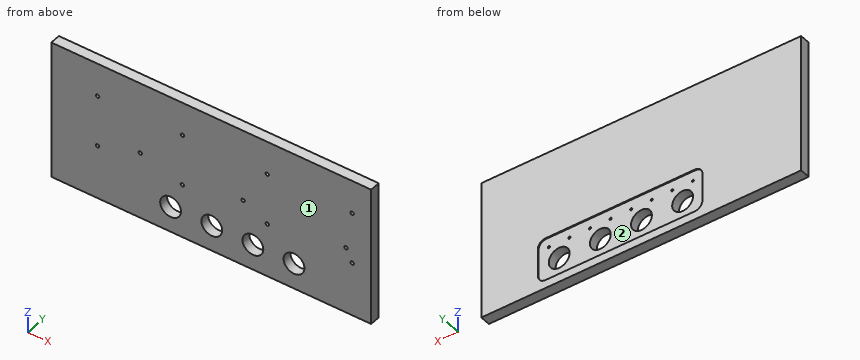
```python
from build123d import *

# Parameters (mm, degrees)
SKETCH_1_W          = 622
SKETCH_1_H          = 270
EXTRUDE_1_DEPTH     = 20
SKETCH_2_W          = 320
SKETCH_2_H          = 84
CUT_EXTRUDE_1_DEPTH = 2
CUT_EXTRUDE_2_REACH = 341.514
SKETCH_3_R          = 20.25
SKETCH_4_R          = 2.1
SKETCH_4_R_2        = 20.25
CUT_EXTRUDE_3_DEPTH = 10
FILLET_1_R          = 15
SKETCH_5_R          = 3.35
CUT_EXTRUDE_4_DEPTH = 12


with BuildPart() as part:
    # 草图1 → 凸台-拉伸1 (new body)
    with BuildSketch(Plane(origin=(0, 0, 0), x_dir=(1, 0, 0), z_dir=(0, 1, 0))):
        Rectangle(SKETCH_1_W, SKETCH_1_H)
    extrude(amount=EXTRUDE_1_DEPTH)

    # 草图2 → 切除-拉伸1 (cut)
    with BuildSketch(Plane(origin=(0, 20, 0), x_dir=(1, 0, 0), z_dir=(0, 1, 0))):
        with Locations((41, 77)):
            Rectangle(SKETCH_2_W, SKETCH_2_H)
    extrude(amount=-CUT_EXTRUDE_1_DEPTH, mode=Mode.SUBTRACT)

    # 草图3 → 切除-拉伸2 (cut, up to next)
    with BuildSketch(Plane(origin=(0, 18, 0), x_dir=(1, 0, 0), z_dir=(0, 1, 0)), mode=Mode.PRIVATE) as cut_extrude_2_sk1:
        with Locations(Location((-79, 85, 0), (0, 0, 270))):
            Circle(SKETCH_3_R)
    cut_extrude_2_tool1 = extrude(cut_extrude_2_sk1.sketch, amount=-CUT_EXTRUDE_2_REACH, mode=Mode.PRIVATE) & part.part
    # 草图3 → 切除-拉伸2 (cut, up to next)
    with BuildSketch(Plane(origin=(0, 18, 0), x_dir=(1, 0, 0), z_dir=(0, 1, 0)), mode=Mode.PRIVATE) as cut_extrude_2_sk2:
        with Locations(Location((1, 85, 0), (0, 0, 270))):
            Circle(SKETCH_3_R)
    cut_extrude_2_tool2 = extrude(cut_extrude_2_sk2.sketch, amount=-CUT_EXTRUDE_2_REACH, mode=Mode.PRIVATE) & part.part
    # 草图3 → 切除-拉伸2 (cut, up to next)
    with BuildSketch(Plane(origin=(0, 18, 0), x_dir=(1, 0, 0), z_dir=(0, 1, 0)), mode=Mode.PRIVATE) as cut_extrude_2_sk3:
        with Locations(Location((81, 85, 0), (0, 0, 270))):
            Circle(SKETCH_3_R)
    cut_extrude_2_tool3 = extrude(cut_extrude_2_sk3.sketch, amount=-CUT_EXTRUDE_2_REACH, mode=Mode.PRIVATE) & part.part
    # 草图3 → 切除-拉伸2 (cut, up to next)
    with BuildSketch(Plane(origin=(0, 18, 0), x_dir=(1, 0, 0), z_dir=(0, 1, 0)), mode=Mode.PRIVATE) as cut_extrude_2_sk4:
        with Locations(Location((161, 85, 0), (0, 0, 270))):
            Circle(SKETCH_3_R)
    cut_extrude_2_tool4 = extrude(cut_extrude_2_sk4.sketch, amount=-CUT_EXTRUDE_2_REACH, mode=Mode.PRIVATE) & part.part
    add(cut_extrude_2_tool1.solids().sort_by_distance((-79, 18, -85))[0], mode=Mode.SUBTRACT)
    add(cut_extrude_2_tool2.solids().sort_by_distance((1, 18, -85))[0], mode=Mode.SUBTRACT)
    add(cut_extrude_2_tool3.solids().sort_by_distance((81, 18, -85))[0], mode=Mode.SUBTRACT)
    add(cut_extrude_2_tool4.solids().sort_by_distance((161, 18, -85))[0], mode=Mode.SUBTRACT)

    # 草图4 → 切除-拉伸3 (cut)
    with BuildSketch(Plane(origin=(0, 18, 0), x_dir=(1, 0, 0), z_dir=(0, 1, 0))):
        with Locations(Location((-99, 54, 0), (0, 0, 270))):
            Circle(SKETCH_4_R)
        with Locations(Location((-79, 85, 0), (0, 0, 270))):
            Circle(SKETCH_4_R_2)
        with Locations(Location((-59, 54, 0), (0, 0, 270))):
            Circle(SKETCH_4_R)
        with Locations(Location((-19, 54, 0), (0, 0, 270))):
            Circle(SKETCH_4_R)
        with Locations(Location((21, 54, 0), (0, 0, 270))):
            Circle(SKETCH_4_R)
        with Locations(Location((61, 54, 0), (0, 0, 270))):
            Circle(SKETCH_4_R)
        with Locations(Location((101, 54, 0), (0, 0, 270))):
            Circle(SKETCH_4_R)
        with Locations(Location((141, 54, 0), (0, 0, 270))):
            Circle(SKETCH_4_R)
        with Locations(Location((181, 54, 0), (0, 0, 270))):
            Circle(SKETCH_4_R)
    extrude(amount=-CUT_EXTRUDE_3_DEPTH, mode=Mode.SUBTRACT)

    # 圆角1
    fillet_1_edges = [part.edges().sort_by_distance(p)[0] for p in [
        (-119, 19, -35),
        (-119, 19, -119),
        (201, 19, -119),
        (201, 19, -35),
    ]]
    fillet(fillet_1_edges, radius=FILLET_1_R)

    # 草图5 → 切除-拉伸4 (cut)
    with BuildSketch(Plane.XZ):
        with Locations(Location((274, -30, 0), (0, 0, 270))):
            Circle(SKETCH_5_R)
        with Locations(Location((262, -5, 0), (0, 0, 270))):
            Circle(SKETCH_5_R)
        with Locations(Location((109, -30, 0), (0, 0, 270))):
            Circle(SKETCH_5_R)
        with Locations(Location((-56, -30, 0), (0, 0, 270))):
            Circle(SKETCH_5_R)
        with Locations(Location((-221, -30, 0), (0, 0, 270))):
            Circle(SKETCH_5_R)
        with Locations(Location((-138, -5, 0), (0, 0, 270))):
            Circle(SKETCH_5_R)
        with Locations(Location((62, -5, 0), (0, 0, 270))):
            Circle(SKETCH_5_R)
        with Locations(Location((274, 70, 0), (0, 0, 270))):
            Circle(SKETCH_5_R)
        with Locations(Location((109, 70, 0), (0, 0, 270))):
            Circle(SKETCH_5_R)
        with Locations(Location((-56, 70, 0), (0, 0, 270))):
            Circle(SKETCH_5_R)
        with Locations(Location((-221, 70, 0), (0, 0, 270))):
            Circle(SKETCH_5_R)
    extrude(amount=-CUT_EXTRUDE_4_DEPTH, mode=Mode.SUBTRACT)


solid = part.part
```
Check sheet for the modelled part. Datum: model origin and axes. Units: mm. Face numbers are marked on the shaded views. Coordinates: 2 decimals unless noted, no trailing zeros. Write each loop counter-clockwise with the first axis right and the second up, starting at its lowest first coordinate (ties: lowest second). Pieces come first, ordered by that corner, then holes. Notation, with made-up numbers: M 38,51.25 L 55,51.25 A17 cw 55,74.25 Z; hole C 51,63.5 d8. An arc over 180 degrees is marked long. Use one line per item in the form item = value.
Item 1: Material ranges on L1, parallel to X at y = 7.5, z = 70; L2, parallel to Z at x = -221, y = 6.75; L3, parallel to X at y = 13.5, z = -85, recorded low to high. Write a range as from..to.
Answer below:
L1 = -311..-224.35, -217.65..-59.35, -52.65..105.65, 112.35..270.65, 277.35..311
L2 = -135..-33.35, -26.65..66.65, 73.35..135
L3 = -311..-99.25, -58.75..-19.25, 21.25..60.75, 101.25..140.75, 181.25..311
Item 2: Sectioned sample at A-A, the plane x = 161. Record the cut outline in (y, z).
Answer below:
outline = M 0,-135 L 20,-135 L 20,-119 L 18,-119 L 18,-105.25 L 0,-105.25 Z; M 0,-64.75 L 18,-64.75 L 18,-35 L 20,-35 L 20,135 L 0,135 Z
Item 3: Sectioned sample at B-B, the plane x = -40.5. Record the cut outline in (y, z).
Answer below:
outline = M 0,-135 L 20,-135 L 20,-119 L 18,-119 L 18,-35 L 20,-35 L 20,135 L 0,135 Z
Item 4: Release check for a two-part mould opening along Z. For the marked faces 1 and 2 record: pulls with the +Z half, pulls with the -Z half, needs draft (parallel to the pull), parting line crosses it, or undercut.
Answer below:
face_1 = needs draft
face_2 = undercut
Item 5: Gauge pin test, flat ends, axial feed: pin 1 Ø1.3 at (x, z) = (-19, -55) entering from +Y; pin 2 Ø2 at (x, z) = (-55.5, 70.5) entering from -Y. Record the tip position at first contact, or that the pin passes through.
Answer below:
pin_1 = 8
pin_2 = 12
